The model under review builds one solid part; all positions refer to its coordinate system, in mm. A direction names the side the tool comes from. Round coordinates to 2 decimals unless told otherwise and drop trailing zeros. Write each loop counter-clockwise with the first axis right and the second up, starting at its lowest first coordinate (ties: lowest second). Pieces come first, ordered by that corner, then holes. Notation, with made-up numbers: M -31,-29 L -23,-29 A26 cw -23,-13 Z; hole C 36,36 d11. An arc over 180 degrees is marked long. Write item = value, one per line. Start each with the question number.
Item 1: Take a section at C-C, the plane y = -3. Give the number of separate pieces and of enclosed holes in the cut face, plus the area to 3 significant figures.
Item 2: Take a section at D-D, the plane x = 15. Give the boundary of the cut face in (y, z), plus the area to 3 significant figures.
Item 3: The part is to be moulded in two halves that separate along X. For faces 5 (the flat face through (-20, -2, -7)), 6 (the flat face through (22.5, -7, 2)), 7 (the flat face through (16.5, -2, -3)), 8 (the cylindrical face through (-25.435, -2.528, 1.946)), say which applies: +X half, -X half, draft (parallel to the pull), parting line (faces both ways), or undercut.
Item 4: For pin 1 Ø2.5 at (y, z) = (5, 1.5) entering from -X; pin 2 Ø6 at (y, z) = (3, -0.5) entering from -X; pin 3 Ø12.5 at (x, y) = (4.5, -4.5) entering from -Z; pin 4 Ø2.5 at (y, z) = (2.5, 2.5) entering from +X, all flat-tipped, find the tip position at first contact; note any pin that passes through.
Item 5: Take a section at A-A, the plane x = -26.5. Give the boundary of the cut face in (y, z).
Item 6: Take a section at B-B, the plane z = -4. Give the boundary of the cut face in (x, y), plus the area to 3 significant figures.
Item 7: To check wall thickness, follow line 1 along X through (y, z) = (-3.7, -4); line 2 along X through (y, z) = (-1.8, 2.5); line 3 along Z through (x, y) = (26.5, -3.4). State the ranges of each line that lie inside material, in increasing order.
Item 8: Tool access review of faces 1 (the flat face through (18.5, 0, 4)), 2 (the flat face through (20.2, -4.5, -2.7)), 3 (the flat face through (-25, -4.5, 3)), 4 (the flat face through (-12.75, 0, 1)): name each direction out of +Z, -Z, +X, -X, +Y, -Y from which nothing blocks a thin tool from reaching the whole face with its end or side.
from build123d import *

# Parameters (mm, degrees)
SKETCH1_W                                       = 45
SKETCH1_H                                       = 25
BOSS_EXTRUDE1_DEPTH                             = 5
SKETCH2_W                                       = 37
SKETCH2_H                                       = 19
CUT_EXTRUDE1_DEPTH                              = 3
FILLET1_R                                       = 2
CUT_EXTRUDE2_DEPTH                              = 26.91331704
FILLET2_R                                       = 4
SKETCH4_W                                       = 5
SKETCH4_H                                       = 5
BOSS_EXTRUDE2_DEPTH                             = 7
CSK_FOR_M2_FLAT_HEAD_MACHINE_SCREW1_D           = 2.4
CSK_FOR_M2_FLAT_HEAD_MACHINE_SCREW1_CSINK_D     = 4.4
CSK_FOR_M2_FLAT_HEAD_MACHINE_SCREW1_CSINK_ANGLE = 90
FILLET3_R                                       = 1
FILLET3_OF_MIRROR1_R                            = 1
SKETCH8_W                                       = 6
SKETCH8_H                                       = 5
BOSS_EXTRUDE3_DEPTH                             = 7
CSK_FOR_M2_FLAT_HEAD_MACHINE_SCREW2_D           = 2.4
CSK_FOR_M2_FLAT_HEAD_MACHINE_SCREW2_CSINK_D     = 4.4
CSK_FOR_M2_FLAT_HEAD_MACHINE_SCREW2_CSINK_ANGLE = 90
FILLET4_R                                       = 1
FILLET4_OF_MIRROR2_R                            = 1


with BuildPart() as part:
    # Sketch1 → Boss-Extrude1 (new body)
    with BuildSketch(Plane.XY):
        Rectangle(SKETCH1_W, SKETCH1_H)
    extrude(amount=BOSS_EXTRUDE1_DEPTH)

    # Sketch2 → Cut-Extrude1 (cut)
    with BuildSketch(Plane.XY.offset(5)):
        Rectangle(SKETCH2_W, SKETCH2_H)
    extrude(amount=-CUT_EXTRUDE1_DEPTH, mode=Mode.SUBTRACT)

    # Fillet1
    fillet1_edges = [part.edges().sort_by_distance(p)[0] for p in [
        (18.5, 9.5, 3.5),
        (18.5, -9.5, 3.5),
        (-18.5, -9.5, 3.5),
        (-18.5, 9.5, 3.5),
    ]]
    fillet(fillet1_edges, radius=FILLET1_R)

    # Sketch3 → Cut-Extrude2 (cut, through all)
    with BuildSketch(Plane.XY.offset(2)):
        with BuildLine():
            Line((-10.75, -3.75), (10.75, -3.75))
            ThreePointArc((10.75, -3.75), (12.164213562, -3.164213562), (12.75, -1.75))
            Line((12.75, -1.75), (12.75, 1.75))
            ThreePointArc((12.75, 1.75), (12.164213562, 3.164213562), (10.75, 3.75))
            Line((10.75, 3.75), (-10.75, 3.75))
            ThreePointArc((-10.75, 3.75), (-12.164213562, 3.164213562), (-12.75, 1.75))
            Line((-12.75, 1.75), (-12.75, -1.75))
            ThreePointArc((-12.75, -1.75), (-12.164213562, -3.164213562), (-10.75, -3.75))
        make_face()
    extrude(amount=-CUT_EXTRUDE2_DEPTH, mode=Mode.SUBTRACT)

    # Fillet2
    fillet2_edges = [part.edges().sort_by_distance(p)[0] for p in [
        (22.5, -12.5, 2.5),
        (-22.5, -12.5, 2.5),
        (-22.5, 12.5, 2.5),
        (22.5, 12.5, 2.5),
    ]]
    fillet(fillet2_edges, radius=FILLET2_R)

    # Sketch4 → Boss-Extrude2 (add)
    with BuildSketch(Plane(origin=(22.5, 0, 0), x_dir=(0, 0, -1), z_dir=(1, 0, 0))):
        with Locations((-2.5, -2)):
            Rectangle(SKETCH4_W, SKETCH4_H)
    boss_extrude2 = extrude(amount=BOSS_EXTRUDE2_DEPTH)

    # CSK for M2 Flat Head Machine Screw1 (through all)
    with Locations(Plane(origin=(26.5, 0.5, 2.5), x_dir=(0, 0, 1), z_dir=(0, 1, 0))):
        with Locations((0, 0)):
            csk_for_m2_flat_head_machine_screw1 = CounterSinkHole(CSK_FOR_M2_FLAT_HEAD_MACHINE_SCREW1_D / 2, CSK_FOR_M2_FLAT_HEAD_MACHINE_SCREW1_CSINK_D / 2, counter_sink_angle=CSK_FOR_M2_FLAT_HEAD_MACHINE_SCREW1_CSINK_ANGLE)

    # Fillet3
    fillet3_edges = [part.edges().sort_by_distance(p)[0] for p in [
        (29.5, -2, 5),
        (29.5, -2, 0),
    ]]
    fillet(fillet3_edges, radius=FILLET3_R)

    # Mirror1: Boss-Extrude2, CSK for M2 Flat Head Machine Screw1 across plane
    add(boss_extrude2.mirror(Plane(origin=(0, 0, 0), x_dir=(0, 0, 1), z_dir=(1, 0, 0))))
    add(csk_for_m2_flat_head_machine_screw1.mirror(Plane(origin=(0, 0, 0), x_dir=(0, 0, 1), z_dir=(1, 0, 0))), mode=Mode.SUBTRACT)

    # Fillet3 of Mirror1
    fillet3_of_mirror1_edges = [part.edges().sort_by_distance(p)[0] for p in [
        (-29.5, -2, 5),
        (-29.5, -2, 0),
    ]]
    fillet(fillet3_of_mirror1_edges, radius=FILLET3_OF_MIRROR1_R)

    # Sketch8 → Boss-Extrude3 (add)
    with BuildSketch(Plane(origin=(0, 0, 0), x_dir=(-1, 0, 0), z_dir=(0, 0, -1))):
        with Locations((-19.5, -2)):
            Rectangle(SKETCH8_W, SKETCH8_H)
    boss_extrude3 = extrude(amount=BOSS_EXTRUDE3_DEPTH)

    # CSK for M2 Flat Head Machine Screw2 (through all)
    with Locations(Plane(origin=(19.5, 0.5, -4), x_dir=(0, 0, 1), z_dir=(0, 1, 0))):
        with Locations((0, 0)):
            csk_for_m2_flat_head_machine_screw2 = CounterSinkHole(CSK_FOR_M2_FLAT_HEAD_MACHINE_SCREW2_D / 2, CSK_FOR_M2_FLAT_HEAD_MACHINE_SCREW2_CSINK_D / 2, counter_sink_angle=CSK_FOR_M2_FLAT_HEAD_MACHINE_SCREW2_CSINK_ANGLE)

    # Fillet4
    fillet4_edges = [part.edges().sort_by_distance(p)[0] for p in [
        (22.5, -2, -7),
        (16.5, -2, -7),
    ]]
    fillet(fillet4_edges, radius=FILLET4_R)

    # Mirror2: Boss-Extrude3, CSK for M2 Flat Head Machine Screw2 across plane
    add(boss_extrude3.mirror(Plane(origin=(0, 0, 0), x_dir=(0, 0, 1), z_dir=(1, 0, 0))))
    add(csk_for_m2_flat_head_machine_screw2.mirror(Plane(origin=(0, 0, 0), x_dir=(0, 0, 1), z_dir=(1, 0, 0))), mode=Mode.SUBTRACT)

    # Fillet4 of Mirror2
    fillet4_of_mirror2_edges = [part.edges().sort_by_distance(p)[0] for p in [
        (-22.5, -2, -7),
        (-16.5, -2, -7),
    ]]
    fillet(fillet4_of_mirror2_edges, radius=FILLET4_OF_MIRROR2_R)


solid = part.part
Response values:
q1.separate_pieces = 2
q1.enclosed_holes = 4
q1.area = 199 mm2
q2.outline = M -12.5,0 L 12.5,0 L 12.5,5 L 9.5,5 L 9.5,2 L -9.5,2 L -9.5,5 L -12.5,5 Z
q2.area = 68.0 mm2
q3.face_5 = draft
q3.face_6 = +X half
q3.face_7 = undercut
q3.face_8 = undercut
q4.pin_1 = -22.5
q4.pin_2 = -29.5
q4.pin_3 = 0
q4.pin_4 = 22.5
q5.outline = M -4.5,0 L 0.5,0 L 0.5,0.3 L -0.5,1.3 L -4.5,1.3 Z; M -4.5,3.7 L -0.5,3.7 L 0.5,4.7 L 0.5,5 L -4.5,5 Z
q6.outline = M -22.5,-4.5 L -20.7,-4.5 L -20.7,-0.5 L -21.7,0.5 L -22.5,0.5 Z; M -18.3,-4.5 L -16.5,-4.5 L -16.5,0.5 L -17.3,0.5 L -18.3,-0.5 Z; M 16.5,-4.5 L 18.3,-4.5 L 18.3,-0.5 L 17.3,0.5 L 16.5,0.5 Z; M 20.7,-4.5 L 22.5,-4.5 L 22.5,0.5 L 21.7,0.5 L 20.7,-0.5 Z
q6.area = 34.0 mm2
q7.line_1 = -22.5 to -20.7, -18.3 to -16.5, 16.5 to 18.3, 20.7 to 22.5
q7.line_2 = -29.5 to -27.7, -25.3 to -18.5, 18.5 to 25.3, 27.7 to 29.5
q7.line_3 = 0 to 1.3, 3.7 to 5
q8.face_1 = +Z
q8.face_2 = -Z, +X, -X, -Y
q8.face_3 = +Z, -Z, -X, -Y
q8.face_4 = +Z, -Z
